The model under review builds one solid part; all positions refer to its coordinate system, in mm. A direction names the side the tool comes from. Give positions to 0.01 mm unless a question says otherwise; leave off trailing zeros. Write each loop counter-clockwise with the first axis right and the second up, starting at its lowest first coordinate (ties: lowest second). Pieces come first, ordered by that corner, then holes.
from build123d import *

# Parameters (mm, degrees)
BOSS_EXTRUDE2_DEPTH = 30


with BuildPart() as part:
    # Sketch1 → Boss-Extrude2 (new body)
    with BuildSketch(Plane.XY):
        with BuildLine():
            Line((-30, 17.5), (-20, 17.5))
            Line((-20, 17.5), (-20, 7.5))
            Line((-20, 7.5), (-10, 7.5))
            ThreePointArc((-10, 7.5), (0, -2.5), (10, 7.5))
            Line((10, 7.5), (20, 7.5))
            Line((20, 7.5), (20, 17.5))
            Line((20, 17.5), (29.681023884, 17.5))
            Line((29.681023884, 17.5), (29.681023884, 16.984704446))
            Line((29.681023884, 16.984704446), (29.681023884, -17.5))
            Line((29.681023884, -17.5), (-30, -17.5))
            Line((-30, -17.5), (-30, 16.984704446))
            Line((-30, 16.984704446), (-30, 17.5))
        make_face()
    extrude(amount=BOSS_EXTRUDE2_DEPTH)


solid = part.part
1) Insertion check: pin 1 (8 mm diameter, centred on x = 13.5, z = 15.5, fed in from +Y); pin 2 (2 mm diameter, centred on x = 6.5, y = 2.5, fed in from -Z). Each pin has a flat end and moves straight along its axis. Give the tip position at first contact, or say it passes through.
2) The part is to be moulded in two halves that separate along X. For faces 3 (the flat face through (0, -4, 30)), 4 (the flat face through (29.681, 0, 15)), 5 (the flat face through (15, 7.5, 15)), say which applies: +X half, -X half, draft (parallel to the pull), parting line (faces both ways), or undercut.
3) Consider section B-B, the plane z = 24.75. Give the boundary of the cut face in (x, y).
4) Consider section D-D, the plane x = 16. Give the boundary of the cut face in (y, z), then the cut area to 3 significant figures.
5) Tool access review of faces 1 (the flat face through (20, 12, 15)), 2 (the flat face through (0, -4, 0)): name each direction out of +Z, -Z, +X, -X, +Y, -Y from which nothing blocks a thin tool from reaching the whole face with its end or side.
6) To check wall thickness, follow probe 1 along X at (y, z) = (10.5, 21); probe 2 along Y at (x, z) = (-11.5, 6.25); probe 3 along X at (y, z) = (3, 8.5). State the ranges of each line that lie inside material, in increasing order.
7) Consider section A-A, the plane y = 11. Give the boundary of the cut face in (x, z).
8) Consider section C-C, the plane x = 0. Give the boundary of the cut face in (y, z).
Answer block:
1. pin 1: stops at y = 7.5
1. pin 2: passes through
2. face 3: draft
2. face 4: +X half
2. face 5: undercut
3. outline: (-30, -17.5) - (29.68, -17.5) - (29.68, 17.5) - (20, 17.5) - (20, 7.5) - (10, 7.5) arc R10 cw to (-10, 7.5) - (-20, 7.5) - (-20, 17.5) - (-30, 17.5) - close
4. outline: (-17.5, 0) - (7.5, 0) - (7.5, 30) - (-17.5, 30) - close
4. area: 750 mm2
5. face 1: +Z, -Z, +Y
5. face 2: -Z, +X, -X, +Y, -Y
6. probe 1: x = -30 to -20, 20 to 29.68
6. probe 2: y = -17.5 to 7.5
6. probe 3: x = -30 to -8.93, 8.93 to 29.68
7. outline: (-30, 0) - (-20, 0) - (-20, 30) - (-30, 30) - close; (20, 0) - (29.68, 0) - (29.68, 30) - (20, 30) - close
8. outline: (-17.5, 0) - (-2.5, 0) - (-2.5, 30) - (-17.5, 30) - close
